Design review of the part built by this model. Coordinates are the model's own, in mm. A direction names the side the tool comes from. Coordinates: 2 decimals unless noted, no trailing zeros. Write each loop counter-clockwise with the first axis right and the second up, starting at its lowest first coordinate (ties: lowest second). Pieces come first, ordered by that corner, then holes. Notation, with made-up numbers: (84.5, 0) - (118.5, 0) arc R34 ccw to (118.5, 36) - close; hole circle Ø11 at (86.5, 52). An arc over 180 degrees is marked (long way). Answer as a JSON object with one key per item and string values.
```python
from build123d import *

# Parameters (mm, degrees)
EXTRUDE_3_DEPTH     = 1.5
EXTRUDE_4_DEPTH     = 13.5
CUT_EXTRUDE_2_DEPTH = 0.4
FILLET_2_R          = 0.2
CUT_EXTRUDE_3_DEPTH = 0.4


with BuildPart() as part:
    # 草图1 → 凸台-拉伸3 (new body)
    with BuildSketch(Plane.XY):
        with BuildLine():
            Line((-5.371727749, 2.046879183), (6.628272251, 2.046879183))
            ThreePointArc((6.628272251, 2.046879183), (8.128272251, 0.546879183), (6.628272251, -0.953120817))
            Line((6.628272251, -0.953120817), (-5.371727749, -0.953120817))
            ThreePointArc((-5.371727749, -0.953120817), (-6.871727749, 0.546879183), (-5.371727749, 2.046879183))
        make_face()
    extrude(amount=EXTRUDE_3_DEPTH)

    # 草图2 → 凸台-拉伸4 (add)
    with BuildSketch(Plane.XY.offset(1.5)):
        Polygon((-5.371727749, -0.07294571), (-5.371727749, 0.22705429), (6.628272251, 0.22705429), (6.628272251, -0.07294571), (6.628272251, -0.47294571), (-5.371727749, -0.47294571), align=None)
    extrude(amount=EXTRUDE_4_DEPTH)

    # 草图3 → 切除-拉伸2 (cut)
    with BuildSketch(Plane(origin=(0, 0.22705429, 0), x_dir=(1, 0, 0), z_dir=(0, 1, 0))):
        Polygon((-2.871727749, -4.5), (-2.871727749, -12.5), (3.128272251, -12.5), (3.128272251, -5.1), (1.784565104, -4.5), align=None)
    extrude(amount=-CUT_EXTRUDE_2_DEPTH, mode=Mode.SUBTRACT)

    # 圆角2
    fillet_2_edges = [part.edges().sort_by_distance(p)[0] for p in [
        (0.628272251, 0.22705429, 1.5),
        (6.628272251, 0.22705429, 8.25),
        (-5.371727749, -0.12294571, 1.5),
        (-5.371727749, 0.22705429, 8.25),
        (0.628272251, -0.47294571, 1.5),
        (-5.371727749, -0.47294571, 8.25),
        (6.628272251, -0.12294571, 1.5),
        (6.628272251, -0.47294571, 8.25),
        (6.628272251, -0.12294571, 15),
        (0.628272251, 0.22705429, 15),
        (-5.371727749, -0.12294571, 15),
        (0.628272251, -0.47294571, 15),
    ]]
    fillet(fillet_2_edges, radius=FILLET_2_R)

    # 草图4 → 切除-拉伸3 (cut)
    with BuildSketch(Plane(origin=(0, 0.22705429, 0), x_dir=(1, 0, 0), z_dir=(0, 1, 0))):
        Polygon((-2.871727749, -12.5), (-2.871727749, -4.5), (2.328272251, -4.5), (3.128272251, -5.1), (3.128272251, -12.5), align=None)
    extrude(amount=-CUT_EXTRUDE_3_DEPTH, mode=Mode.SUBTRACT)


solid = part.part
```
(1) The part is to be moulded in two halves that separate along Z. For faces 1 (the face through (0, -0.173, 8)), 2 (the face through (1, 1, 0)), 3 (the face through (1, -0.473, 8)), say which applies: pulls with the +Z half, pulls with the -Z half, needs draft (parallel to the pull), parting line crosses it, or undercut.
Solved:
{"face 1": "undercut", "face 2": "pulls with the -Z half", "face 3": "needs draft"}
(2) Take a section at A-A, the plane z = 14. Write out the cut boundary in (x, y).
Solved:
{"outline": "(-5.37, -0.27) arc R0.2 ccw to (-5.17, -0.47) - (6.43, -0.47) arc R0.2 ccw to (6.63, -0.27) - (6.63, 0.03) arc R0.2 ccw to (6.43, 0.23) - (-5.17, 0.23) arc R0.2 ccw to (-5.37, 0.03) - close"}
(3) Take a section at C-C, the plane z = 6.5. Write out the cut boundary in (x, y).
Solved:
{"outline": "(-5.37, -0.27) arc R0.2 ccw to (-5.17, -0.47) - (6.43, -0.47) arc R0.2 ccw to (6.63, -0.27) - (6.63, 0.03) arc R0.2 ccw to (6.43, 0.23) - (3.13, 0.23) - (3.13, -0.17) - (-2.87, -0.17) - (-2.87, 0.23) - (-5.17, 0.23) arc R0.2 ccw to (-5.37, 0.03) - close"}
(4) Tool access review of faces 4 (the face through (1, 2.047, 1)), 5 (the face through (4, 0.227, 8)): name each direction out of +Z, -Z, +X, -X, +Y, -Y from which nothing blocks a thin tool from reaching the whole face with its end or side.
Solved:
{"face 4": "+Z, -Z, +X, -X, +Y", "face 5": "+Z, +X, -X, +Y"}
(5) For pin 1 (4 mm diameter, centred on x = 4, z = 5, fed in from +Y); pin 2 (1.8 mm diameter, centred on x = -1, z = 10, fed in from +Y); pin 3 (3 mm diameter, centred on x = -2, z = 7, fed in from -Y), all flat-tipped, find the tip position at first contact; note any pin that passes through.
Solved:
{"pin 1": "stops at y = 0.23", "pin 2": "stops at y = -0.17", "pin 3": "stops at y = -0.47"}
(6) To check wall thickness, follow line 1 (Y direction, x = -3, z = 11); line 2 (Z direction, x = 0.5, y = 0); line 3 (Z direction, x = 5.25, y = 0.4). State the ranges of each line that lie inside material, in increasing order. Write a range as from..to.
Solved:
{"line 1": "y = -0.47..0.23", "line 2": "z = 0..4.5, 12.5..15", "line 3": "z = 0..1.5"}
(7) Take a section at D-D, the plane y = 1.35. Write out the cut boundary in (x, z), and give its area (3 significant figures).
Solved:
{"outline": "(-6.64, 0) - (7.9, 0) - (7.9, 1.5) - (-6.64, 1.5) - close", "area": "21.8 mm^2"}
(8) Take a section at B-B, the plane x = 1.75. Write out the cut boundary in (y, z), and give its area (4 significant figures).
Solved:
{"outline": "(-0.95, 0) - (2.05, 0) - (2.05, 1.5) - (0.43, 1.5) arc R0.2 cw to (0.23, 1.7) - (0.23, 4.5) - (-0.17, 4.5) - (-0.17, 12.5) - (0.23, 12.5) - (0.23, 14.8) arc R0.2 ccw to (0.03, 15) - (-0.27, 15) arc R0.2 ccw to (-0.47, 14.8) - (-0.47, 1.7) arc R0.2 cw to (-0.67, 1.5) - (-0.95, 1.5) - close", "area": "10.75 mm^2"}
